```python
from build123d import *

# Parameters (mm, degrees)
F0_W     = 200
F0_H     = 400
F0_W_2   = 60
F0_H_2   = 12
F1_DEPTH = 20
F2_D     = 4.4
F3_R     = 5


with BuildPart() as f1:
    # F0 (on Top) → F1 (new body)
    with BuildSketch(Plane.XY):
        Rectangle(F0_W, F0_H)
        with Locations((-45, 131)):
            Rectangle(F0_W_2, F0_H_2, mode=Mode.SUBTRACT)
        with Locations((45, 131)):
            Rectangle(F0_W_2, F0_H_2, mode=Mode.SUBTRACT)
    extrude(amount=F1_DEPTH)

    # F2 (through all)
    with Locations(Plane(origin=(0, 0, 0), x_dir=(1, 0, 0), z_dir=(0, 0, -1))):
        with Locations((-26.5, -155), (26.5, -155), (-66, 59), (-24, 59), (24, 59), (66, 59), (-66, -155), (-66, -145), (66, -155), (66, -145), (-29, 44), (29, 44), (-30, 195), (30, 195), (-60, 41)):
            Hole(F2_D / 2)

    # F3
    f3_edges = [f1.edges().sort_by_distance(p)[0] for p in [
        (-75, 131, 20),
        (-15, 131, 20),
        (15, 131, 20),
        (75, 131, 20),
    ]]
    fillet(f3_edges, radius=F3_R)


solid = f1.part
```
Here's how the part is built. I have some questions about the finished solid (model axes, mm). A direction names the side the tool comes from. Give positions to 0.01 mm unless a question says otherwise; leave off trailing zeros. Loops run counter-clockwise (first coordinate to the right, second up) from the corner with the lowest first, then second, coordinate; pieces in that order, holes last. Notation, with made-up numbers: M 3.25,56 L 41.25,56 A31 ccw 41.25,84 Z; hole C 45.25,74.5 d10. An arc over 180 degrees is marked long. Use one line per item in the form item = value. Start each with the question number.
Q1. If we section it at A-A (x = -48.5): Write out the boundary of the cut face in (y, z).
Q2. If we section it at B-B (z = 11.5): State how many separate pieces and enclosed holes the cut face has, then the cut area to 3 significant figures.
Q3. Will this pin go through, and if not, where does the flat tip stop? pin 1 Ø7 at (x, y) = (29, -44) entering from +Z.
Q4. Thinking about a two-plate mould opening in X: for faces 3 (the flat face through (15, 131, 7)), 4 (the flat face through (-45, 125, 10)), 5 (the flat face through (100, -3, 10)), 6 (the flat face through (-1, 200, 10)), which applies, +X half, -X half, draft (parallel to the pull), parting line (faces both ways), or undercut?
Q5. I need wall thicknesses on line 1 along Y through (x, z) = (-26.5, 14.75); line 2 along X through (y, z) = (155, 10); line 3 along Y through (x, z) = (-66, 15.75). Which ranges of each line are inside material? Lowest first, please.
Q6. Which directions (+Z, -Z, +X, -X, +Y, -Y) give clear straight access to the entire face, cutting with the end or side of a thin tool? Please do faces 1 (the flat face through (-1, 3, 20)), 2 (the flat face through (-75, 131, 7)).
Taken from the geometry:
q1.outline = M -200,0 L 125,0 L 125,20 L -200,20 Z; M 137,0 L 200,0 L 200,20 L 137,20 Z
q2.separate_pieces = 1
q2.enclosed_holes = 17
q2.area = 78,300 mm^2
q3.pin_1 = 20
q4.face_3 = undercut
q4.face_4 = undercut
q4.face_5 = +X half
q4.face_6 = draft
q5.line_1 = -200 to 125, 137 to 152.8, 157.2 to 200
q5.line_2 = -100 to -68.2, -63.8 to -28.7, -24.3 to 24.3, 28.7 to 63.8, 68.2 to 100
q5.line_3 = -200 to -61.2, -56.8 to 125, 137 to 142.8, 147.2 to 152.8, 157.2 to 200
q6.face_1 = +Z, +X, -X, +Y, -Y
q6.face_2 = +Z, -Z
